```python
from build123d import *

# Parameters (mm, degrees)
SKETCH1_W                      = 152.4
SKETCH1_H                      = 101.6
BASE_FLANGE1_DEPTH             = 1.6002
EDGE_FLANGE1_DEPTH             = 152.4
EDGE_FLANGE2_DEPTH             = 152.4
CUT_EXTRUDE1_DEPTH             = 95.949783169
EDGE_FLANGE7_STRIP_W           = 7.874
EDGE_FLANGE7_STRIP_H           = 1.6002
EDGE_FLANGE7_STRIP_CUT_DEPTH   = 152.4
EDGE_FLANGE7_DEPTH             = 152.4
EDGE_FLANGE8_STRIP_W           = 7.874
EDGE_FLANGE8_STRIP_H           = 1.6002
EDGE_FLANGE8_STRIP_CUT_DEPTH   = 152.4
EDGE_FLANGE8_DEPTH             = 152.4
SKETCH35_W                     = 35.56
SKETCH35_H                     = 1.6002
BOSS_EXTRUDE1_DEPTH            = 19.7358
EDGE_FLANGE9_STRIP_W           = 7.874
EDGE_FLANGE9_STRIP_H           = 1.6002
EDGE_FLANGE9_STRIP_CUT_DEPTH   = 35.56
EDGE_FLANGE9_DEPTH             = 35.56
SKETCH39_W                     = 36.50996
SKETCH39_H                     = 1.6002
BOSS_EXTRUDE2_DEPTH            = 19.7358
EDGE_FLANGE10_STRIP_W          = 7.874
EDGE_FLANGE10_STRIP_H          = 1.6002
EDGE_FLANGE10_STRIP_CUT_DEPTH  = 36.50996
EDGE_FLANGE10_DEPTH            = 36.50996
CUT_EXTRUDE2_REACH             = 111.661
SKETCH43_R                     = 3.37312
CUT_EXTRUDE2_DIRECTION_2_REACH = 111.661
FILLET1_R                      = 12.7
SKETCH45_R                     = 5.715
CUT_EXTRUDE3_DEPTH             = 1.6002


# Sheet-metal steps are written as plain solids
with BuildPart() as part:
    # Sketch1 → Base-Flange1 (new body)
    with BuildSketch(Plane.XY):
        Rectangle(SKETCH1_W, SKETCH1_H)
    extrude(amount=-BASE_FLANGE1_DEPTH)

    # Edge-Flange1 section (across the edge) → Edge-Flange1 (add)
    with BuildSketch(Plane(origin=(-76.2, 51.5366, -1.6002), x_dir=(0, -1, 0), z_dir=(1, 0, 0))):
        with BuildLine():
            Line((-1.6002, 0.7366), (-1.6002, 18.034))
            Line((-1.6002, 18.034), (0, 18.034))
            Line((0, 18.034), (0, 0.7366))
            ThreePointArc((0, 0.7366), (0.215745145, 0.215745145), (0.7366, 0))
            Line((0.7366, 0), (0.7366, -1.6002))
            ThreePointArc((0.7366, -1.6002), (-0.915767126, -0.915767126), (-1.6002, 0.7366))
        make_face()
    extrude(amount=EDGE_FLANGE1_DEPTH)

    # Edge-Flange2 section (across the edge) → Edge-Flange2 (add)
    with BuildSketch(Plane(origin=(76.2, -51.5366, -1.6002), x_dir=(0, 1, 0), z_dir=(-1, 0, 0))):
        with BuildLine():
            Line((-1.6002, 0.7366), (-1.6002, 18.034))
            Line((-1.6002, 18.034), (0, 18.034))
            Line((0, 18.034), (0, 0.7366))
            ThreePointArc((0, 0.7366), (0.215745145, 0.215745145), (0.7366, 0))
            Line((0.7366, 0), (0.7366, -1.6002))
            ThreePointArc((0.7366, -1.6002), (-0.915767126, -0.915767126), (-1.6002, 0.7366))
        make_face()
    extrude(amount=EDGE_FLANGE2_DEPTH)

    # Sketch14 → Cut-Extrude1 (cut, through all)
    with BuildSketch(Plane.XY):
        Polygon((76.2, -38.1), (76.2, 38.1), (38.1, 38.1), (38.1, -23.241), (15.24, -23.241), (15.24, -38.1), align=None)
    extrude(amount=-CUT_EXTRUDE1_DEPTH, mode=Mode.SUBTRACT)

    # Edge-Flange7 strip (across the edge) → Edge-Flange7 strip cut (cut)
    with BuildSketch(Plane(origin=(76.2, -51.5366, -19.6342), x_dir=(0, 0, 1), z_dir=(-1, 0, 0))):
        with Locations((-1.6002, -0.8001)):
            Rectangle(EDGE_FLANGE7_STRIP_W, EDGE_FLANGE7_STRIP_H)
    extrude(amount=EDGE_FLANGE7_STRIP_CUT_DEPTH, mode=Mode.SUBTRACT)

    # Edge-Flange7 section (across the edge) → Edge-Flange7 (add)
    with BuildSketch(Plane(origin=(76.2, -51.5366, -19.6342), x_dir=(0, 0, 1), z_dir=(-1, 0, 0))):
        with BuildLine():
            Line((0, 0.7366), (0, 8.5598))
            Line((0, 8.5598), (1.6002, 8.5598))
            Line((1.6002, 8.5598), (1.6002, 0.7366))
            ThreePointArc((1.6002, 0.7366), (1.815945145, 0.215745145), (2.3368, 0))
            Line((2.3368, 0), (2.3368, -1.6002))
            ThreePointArc((2.3368, -1.6002), (0.684432874, -0.915767126), (0, 0.7366))
        make_face()
    extrude(amount=EDGE_FLANGE7_DEPTH)

    # Edge-Flange8 strip (across the edge) → Edge-Flange8 strip cut (cut)
    with BuildSketch(Plane(origin=(-76.2, 51.5366, -19.6342), x_dir=(0, 0, 1), z_dir=(1, 0, 0))):
        with Locations((-1.6002, -0.8001)):
            Rectangle(EDGE_FLANGE8_STRIP_W, EDGE_FLANGE8_STRIP_H)
    extrude(amount=EDGE_FLANGE8_STRIP_CUT_DEPTH, mode=Mode.SUBTRACT)

    # Edge-Flange8 section (across the edge) → Edge-Flange8 (add)
    with BuildSketch(Plane(origin=(-76.2, 51.5366, -19.6342), x_dir=(0, 0, 1), z_dir=(1, 0, 0))):
        with BuildLine():
            Line((0, 0.7366), (0, 8.5598))
            Line((0, 8.5598), (1.6002, 8.5598))
            Line((1.6002, 8.5598), (1.6002, 0.7366))
            ThreePointArc((1.6002, 0.7366), (1.815945145, 0.215745145), (2.3368, 0))
            Line((2.3368, 0), (2.3368, -1.6002))
            ThreePointArc((2.3368, -1.6002), (0.684432874, -0.915767126), (0, 0.7366))
        make_face()
    extrude(amount=EDGE_FLANGE8_DEPTH)

    # Sketch35 → Boss-Extrude1 (add)
    with BuildSketch(Plane(origin=(0, -42.9768, 0), x_dir=(1, 0, 0), z_dir=(0, 1, 0))):
        with Locations((58.42, 18.8341)):
            Rectangle(SKETCH35_W, SKETCH35_H)
    extrude(amount=BOSS_EXTRUDE1_DEPTH)

    # Edge-Flange9 strip (across the edge) → Edge-Flange9 strip cut (cut)
    with BuildSketch(Plane(origin=(76.2, -23.241, -18.034), x_dir=(0, -1, 0), z_dir=(-1, 0, 0))):
        with Locations((-1.6002, -0.8001)):
            Rectangle(EDGE_FLANGE9_STRIP_W, EDGE_FLANGE9_STRIP_H)
    extrude(amount=EDGE_FLANGE9_STRIP_CUT_DEPTH, mode=Mode.SUBTRACT)

    # Edge-Flange9 section (across the edge) → Edge-Flange9 (add)
    with BuildSketch(Plane(origin=(76.2, -23.241, -18.034), x_dir=(0, -1, 0), z_dir=(-1, 0, 0))):
        with BuildLine():
            Line((0, 0.7366), (0, 13.6398))
            Line((0, 13.6398), (1.6002, 13.6398))
            Line((1.6002, 13.6398), (1.6002, 0.7366))
            ThreePointArc((1.6002, 0.7366), (1.815945145, 0.215745145), (2.3368, 0))
            Line((2.3368, 0), (2.3368, -1.6002))
            ThreePointArc((2.3368, -1.6002), (0.684432874, -0.915767126), (0, 0.7366))
        make_face()
    extrude(amount=EDGE_FLANGE9_DEPTH)

    # Sketch39 → Boss-Extrude2 (add)
    with BuildSketch(Plane.XZ.offset(-42.9768)):
        with Locations((57.94502, -18.8341)):
            Rectangle(SKETCH39_W, SKETCH39_H)
    extrude(amount=BOSS_EXTRUDE2_DEPTH)

    # Edge-Flange10 strip (across the edge) → Edge-Flange10 strip cut (cut)
    with BuildSketch(Plane(origin=(39.69004, 23.241, -18.034), x_dir=(0, 1, 0), z_dir=(1, 0, 0))):
        with Locations((-1.6002, -0.8001)):
            Rectangle(EDGE_FLANGE10_STRIP_W, EDGE_FLANGE10_STRIP_H)
    extrude(amount=EDGE_FLANGE10_STRIP_CUT_DEPTH, mode=Mode.SUBTRACT)

    # Edge-Flange10 section (across the edge) → Edge-Flange10 (add)
    with BuildSketch(Plane(origin=(39.69004, 23.241, -18.034), x_dir=(0, 1, 0), z_dir=(1, 0, 0))):
        with BuildLine():
            Line((0, 0.7366), (0, 13.6398))
            Line((0, 13.6398), (1.6002, 13.6398))
            Line((1.6002, 13.6398), (1.6002, 0.7366))
            ThreePointArc((1.6002, 0.7366), (1.815945145, 0.215745145), (2.3368, 0))
            Line((2.3368, 0), (2.3368, -1.6002))
            ThreePointArc((2.3368, -1.6002), (0.684432874, -0.915767126), (0, 0.7366))
        make_face()
    extrude(amount=EDGE_FLANGE10_DEPTH)

    # Cut-Extrude2: up to this face of the body (flat: up to its plane)
    cut_extrude2_end = Plane(part.part.faces().sort_by_distance((58.42, -24.8412, -10.8458))[0])
    # Sketch43 → Cut-Extrude2 (cut, up to the picked face)
    with BuildSketch(Plane(origin=(0, -23.241, 0), x_dir=(1, 0, 0), z_dir=(0, 1, 0)), mode=Mode.PRIVATE) as cut_extrude2_sk1:
        with Locations(Location((57.94502, 10.7442, 0), (0, 0, 270))):
            Circle(SKETCH43_R)
    cut_extrude2_tool1 = split(extrude(cut_extrude2_sk1.sketch, amount=-CUT_EXTRUDE2_REACH, mode=Mode.PRIVATE), bisect_by=cut_extrude2_end, keep=Keep.BOTH, mode=Mode.PRIVATE)
    add(cut_extrude2_tool1.solids().sort_by(Axis((57.94502, -23.241, -10.7442), (0, -1, 0)))[0], mode=Mode.SUBTRACT)

    # Cut-Extrude2 direction 2: up to this face of the body (flat: up to its plane)
    cut_extrude2_direction_2_end = Plane(part.part.faces().sort_by_distance((57.94502, 24.8412, -10.8458))[0])
    # Sketch43 → Cut-Extrude2 direction 2 (cut, up to the picked face)
    with BuildSketch(Plane(origin=(0, -23.241, 0), x_dir=(1, 0, 0), z_dir=(0, 1, 0)), mode=Mode.PRIVATE) as cut_extrude2_direction_2_sk1:
        with Locations(Location((57.94502, 10.7442, 0), (0, 0, 270))):
            Circle(SKETCH43_R)
    cut_extrude2_direction_2_tool1 = split(extrude(cut_extrude2_direction_2_sk1.sketch, amount=CUT_EXTRUDE2_DIRECTION_2_REACH, mode=Mode.PRIVATE), bisect_by=cut_extrude2_direction_2_end, keep=Keep.BOTH, mode=Mode.PRIVATE)
    add(cut_extrude2_direction_2_tool1.solids().sort_by(Axis((57.94502, -23.241, -10.7442), (0, 1, 0)))[0], mode=Mode.SUBTRACT)

    # Fillet1
    fillet1_edges = [part.edges().sort_by_distance(p)[0] for p in [
        (40.64, -42.9768, -18.8341),
        (39.69004, 42.9768, -18.8341),
    ]]
    fillet(fillet1_edges, radius=FILLET1_R)

    # Sketch45 → Cut-Extrude3 (cut)
    with BuildSketch(Plane(origin=(0, 53.1368, 0), x_dir=(1, 0, 0), z_dir=(0, 1, 0))):
        with Locations(Location((57.94502, 10.7442, 0), (0, 0, 270))):
            Circle(SKETCH45_R)
    extrude(amount=-CUT_EXTRUDE3_DEPTH, mode=Mode.SUBTRACT)


solid = part.part
```
Model file for the job. Use its own axes, mm. A direction names the side the tool comes from. Round coordinates to 2 decimals unless told otherwise and drop trailing zeros. Order: outer loops, then holes, each group sorted by start corner. A loop starts at its lowest first (then second) coordinate and runs counter-clockwise, first axis right, second up. Notation, with made-up numbers: (-33.75, 83) -> (10.25, 83) arc R14 cw to (10.25, 109) -> close; hole circle Ø2 at (-29.75, 40). An arc over 180 degrees is marked (long way). Use one line per item in the form item = value.
Item 1: Cut at B-B, the plane z = -9.75. Write the cut outline in (x, y), and give its area (3 significant figures).
Returned:
outline = (-76.2, -53.14) -> (76.2, -53.14) -> (76.2, -51.54) -> (-76.2, -51.54) -> close; (-76.2, 51.54) -> (52.32, 51.54) -> (52.32, 53.14) -> (-76.2, 53.14) -> close; (39.69, 23.24) -> (54.72, 23.24) -> (54.72, 24.84) -> (39.69, 24.84) -> close; (40.64, -24.84) -> (54.72, -24.84) -> (54.72, -23.24) -> (40.64, -23.24) -> close; (61.17, -24.84) -> (76.2, -24.84) -> (76.2, -23.24) -> (61.17, -23.24) -> close; (61.17, 23.24) -> (76.2, 23.24) -> (76.2, 24.84) -> (61.17, 24.84) -> close; (63.57, 51.54) -> (76.2, 51.54) -> (76.2, 53.14) -> (63.57, 53.14) -> close
area = 564 mm^2
Item 2: Cut at A-A, the plane x = 21. Write the cut outline in (y, z).
Returned:
outline = (-53.14, -17.3) arc R2.34 ccw to (-50.8, -19.63) -> (-42.98, -19.63) -> (-42.98, -18.03) -> (-50.8, -18.03) arc R0.74 cw to (-51.54, -17.3) -> (-51.54, -2.34) arc R0.74 cw to (-50.8, -1.6) -> (-38.1, -1.6) -> (-38.1, 0) -> (-50.8, 0) arc R2.34 ccw to (-53.14, -2.34) -> close; (-23.24, -1.6) -> (50.8, -1.6) arc R0.74 cw to (51.54, -2.34) -> (51.54, -17.3) arc R0.74 cw to (50.8, -18.03) -> (42.98, -18.03) -> (42.98, -19.63) -> (50.8, -19.63) arc R2.34 ccw to (53.14, -17.3) -> (53.14, -2.34) arc R2.34 ccw to (50.8, 0) -> (-23.24, 0) -> close
Item 3: Cut at C-C, the plane y = -36.5. Write the cut outline in (x, z), and give its area (3 significant figures).
Returned:
outline = (-76.2, -1.6) -> (15.24, -1.6) -> (15.24, 0) -> (-76.2, 0) -> close; (39.01, -19.63) -> (76.2, -19.63) -> (76.2, -18.03) -> (39.01, -18.03) -> close
area = 206 mm^2
Item 4: Pull direction Z, two halves, no side cores. Call faces 5 (the face through (-18, 1, 0)), 6 (the face through (63.61, 52.35, -11.49)), 7 (the face through (39.69, 24.69, -13.67)): released by +Z, released by -Z, zero draft, split by the parting line, or undercut.
Returned:
face_5 = released by +Z
face_6 = undercut
face_7 = zero draft
Item 5: Flat gauge pins, fed straight in: pin 1 Ø2 at (x, y) = (-27.5, -13) entering from -Z; pin 2 Ø0.5 at (x, z) = (34.5, -1) entering from +Y; pin 3 Ø0.5 at (x, z) = (-10, -19) entering from +Y. Where does each tip first touch, or does it go through?
Returned:
pin_1 = -1.6
pin_2 = 52.87
pin_3 = 52.63
Item 6: Tool access for faces 1 (the face through (16, -44, -18.034)), 2 (the face through (36.821, -39.355, -18.845)), 3 (the face through (63, -23.241, -11)), 4 (the face through (62, 24.841, -11)): list every direction of +Z, -Z, +X, -X, +Y, -Y with a clear straight run to the whole face (end or side of a thin tool).
Returned:
face_1 = +X, -X
face_2 = -Z, -X
face_3 = +Z, -Z, +X, -X
face_4 = +Z, +X, -X
Item 7: Cut at D-D, the plane x = -8. Write the cut outline in (y, z), and give its area (3 significant figures).
Returned:
outline = (-53.14, -17.3) arc R2.34 ccw to (-50.8, -19.63) -> (-42.98, -19.63) -> (-42.98, -18.03) -> (-50.8, -18.03) arc R0.74 cw to (-51.54, -17.3) -> (-51.54, -2.34) arc R0.74 cw to (-50.8, -1.6) -> (50.8, -1.6) arc R0.74 cw to (51.54, -2.34) -> (51.54, -17.3) arc R0.74 cw to (50.8, -18.03) -> (42.98, -18.03) -> (42.98, -19.63) -> (50.8, -19.63) arc R2.34 ccw to (53.14, -17.3) -> (53.14, -2.34) arc R2.34 ccw to (50.8, 0) -> (-50.8, 0) arc R2.34 ccw to (-53.14, -2.34) -> close
area = 251 mm^2
Item 8: Drill centre lines: line 1 (Y direction, x = 65.5, z = -7.5); line 2 (Y direction, x = -52.5, z = -17.25); line 3 (Z direction, x = -2.5, y = -20.5). Where is each one in solid material? Low to high.
Returned:
line_1 = -53.14 to -51.54, -24.84 to -23.24, 23.24 to 24.84, 51.54 to 53.14
line_2 = -53.14 to -51.54, 51.54 to 53.14
line_3 = -1.6 to 0
